Autodesk Inventor part; units mm, degrees
ref_plane "YZ Plane" through (0, 0, 0) normal (1, 0, 0) x (0, 1, 0)
ref_plane "XZ Plane" through (0, 0, 0) normal (0, 1, 0) x (-1, 0, 0)
ref_plane "XY Plane" through (0, 0, 0) normal (0, 0, 1) x (1, 0, 0)
sketch "Sketch1" plane through (0, 0, 0) normal (0, 0, 1) x (1, 0, 0)
  line L0 (0, 0) -> (76.2, 0)
  line L1 (76.2, 0) -> (76.2, 50.8)
  line L2 (76.2, 50.8) -> (0, 50.8)
  line L3 (0, 50.8) -> (0, 0)
  circle A0 centre (18.1795, 25.4) radius 14.2875
  line L4 (76.2, 50.8) -> (57.15, 50.8)
  line L5 (57.15, 39.6875) -> (66.675, 25.4)
  line L6 (66.675, 25.4) -> (57.15, 11.1125)
  dimension "d0" = 76.2
  dimension "d1" = 50.8
  dimension "d2" = 28.575
extrude "Extrusion1" add sketch "Sketch1" along normal blind 6.35
sketch "Sketch2" plane through (0, 0, 6.35) normal (0, 0, 1) x (1, 0, 0)
  line L0 (76.2, 50.8) -> (0, 50.8)
  line L1 (76.2, 50.8) -> (57.15, 50.8)
  line L2 (57.15, 39.6875) -> (66.675, 25.4)
  line L3 (66.675, 25.4) -> (57.15, 11.1125)
hole "Hole1" at (66.675, 25.4, 6.35) at (57.15, 39.6875, 6.35) at (57.15, 11.1125, 6.35) direction (0, 0, -1) diameter 4.7625 end through all
equation "\"d12\" = Thickness"
equation "\"BendRadius\" = Thickness"
equation "\"BendReliefWidth\" = Thickness"
equation "\"BendReliefDepth\" = 0.5 * Thickness"
equation "\"CornerReliefSize\" = 4 * Thickness"
equation "\"MinimumRemnant\" = 2 * Thickness"
equation "\"TransitionRadius\" = BendRadius"
equation "\"JacobiRadiusSize\" = BendRadius"
equation "\"GapSize\" = Thickness"
properties part number "Light Bracket"
Check sheet for the modelled part. Datum: model origin and axes. Units: mm. Coordinates: 2 decimals unless noted, no trailing zeros. Write each loop counter-clockwise with the first axis right and the second up, starting at its lowest first coordinate (ties: lowest second). Pieces come first, ordered by that corner, then holes.
Item 1: Cross-section at A-A on y = 25.4. Record the boundary of the cut face in (x, z), then the cut area to 3 significant figures.
Numbers:
outline: (0, 0) - (3.89, 0) - (3.89, 6.35) - (0, 6.35) - close; (32.47, 0) - (64.29, 0) - (64.29, 6.35) - (32.47, 6.35) - close; (69.06, 0) - (76.2, 0) - (76.2, 6.35) - (69.06, 6.35) - close
area: 272 mm2
Item 2: Depth check by flat-ended pin: pin 1 Ø4.5 at (x, y) = (57.15, 39.69) entering from +Z; pin 2 Ø1.5 at (y, z) = (14.5, 1.5) entering from -X. Enter the tip coordinate at first touch or a pass-through.
Numbers:
pin 1: passes through
pin 2: stops at x = 0
Item 3: Scan lines: probe 1 along Y at (x, z) = (57.15, 2.25); probe 2 along X at (y, z) = (13, 1.5); probe 3 along X at (y, z) = (38.5, 2.25). Record each from-to range of solid material in increasing order.
Numbers:
probe 1: y = 0 to 8.73, 13.49 to 37.31, 42.07 to 50.8
probe 2: x = 0 to 11.08, 25.28 to 55.7, 58.6 to 76.2
probe 3: x = 0 to 12.48, 23.88 to 55.09, 59.21 to 76.2
Item 4: Cross-section at B-B on x = 28. Record the boundary of the cut face in (y, z).
Numbers:
outline: (0, 0) - (15.02, 0) - (15.02, 6.35) - (0, 6.35) - close; (35.78, 0) - (50.8, 0) - (50.8, 6.35) - (35.78, 6.35) - close
Item 5: Cross-section at C-C on x = 57.15. Record the boundary of the cut face in (y, z).
Numbers:
outline: (0, 0) - (8.73, 0) - (8.73, 6.35) - (0, 6.35) - close; (13.49, 0) - (37.31, 0) - (37.31, 6.35) - (13.49, 6.35) - close; (42.07, 0) - (50.8, 0) - (50.8, 6.35) - (42.07, 6.35) - close
Item 6: Mould release check, pull along Y, two halves, no side actions. Record for faces 1 (the face through (38, 0, 3)), 2 (the face through (0, 26, 3)), 3 (the face through (59.475, 11.629, 3.131)): released by +Y, released by -Y, zero draft, split by the parting line, or undercut.
Numbers:
face 1: released by -Y
face 2: zero draft
face 3: undercut
Item 7: Cross-section at D-D on z = 5.5. Count the separate pieces of the cut face and the enclosed holes in it, then the cut area to 3 significant figures.
Numbers:
separate pieces: 1
enclosed holes: 4
area: 3,180 mm2
